The model under review builds one solid part; all positions refer to its coordinate system, in mm. Face numbers are marked on the shaded views. A direction names the side the tool comes from. Round coordinates to 2 decimals unless told otherwise and drop trailing zeros. Write each loop counter-clockwise with the first axis right and the second up, starting at its lowest first coordinate (ties: lowest second). Pieces come first, ordered by that corner, then holes. Notation, with made-up numbers: (86, 16) -> (117, 16) arc R27 ccw to (117, 36) -> close; hole circle Ø1 at (52.25, 34). An arc over 180 degrees is marked (long way). Answer in a Markdown table with one row per item. Add a question column.
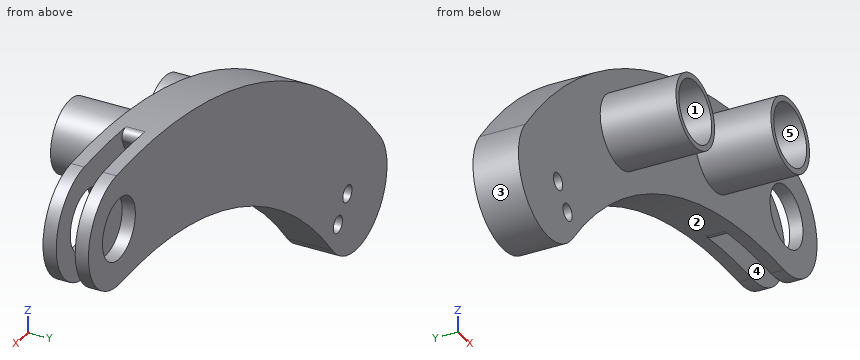
```python
from build123d import *

# Parameters (mm, degrees)
BOSS_EXTRUDE4_DEPTH = 11.999999999999996
BOSS_EXTRUDE5_DEPTH = 3.5
BOSS_EXTRUDE6_DEPTH = 12
CUT_EXTRUDE2_DEPTH  = 8.5
BOSS_EXTRUDE7_DEPTH = 3.5000000000000004
SKETCH2_R           = 8.1
CUT_EXTRUDE3_DEPTH  = 12
FILLET1_R           = 5
FILLET2_R           = 2
SKETCH3_R           = 2.2499999999999964
CUT_EXTRUDE4_DEPTH  = 12
SKETCH4_R           = 9.500000000000002
SKETCH4_R_2         = 8.1
SKETCH4_R_3         = 9.499999999999995
SKETCH4_R_4         = 8.099999999999993
BOSS_EXTRUDE8_DEPTH = 19.999999999999993


with BuildPart() as part:
    # Sketch1 → Boss-Extrude4 (new body)
    with BuildSketch(Plane(origin=(0, 0, 0), x_dir=(1, 0, 0), z_dir=(0, 1, 0))):
        with BuildLine():
            ThreePointArc((-105.23956914411866, 60.05130546378884), (-126.31086817026393, 62.500868149406244), (-128.76043085588134, 41.429569123260976))
            ThreePointArc((-128.76043085588134, 41.42956912326096), (-78.3921989201775, 0.4513014224205847), (-15.424890802752289, -15.400995588922257))
            ThreePointArc((-15.424890802752284, -15.400995588922251), (-20.878753235246265, -0.5691494549701637), (-16.67921047602729, 14.665420305521598))
            ThreePointArc((-16.679210476027265, 14.665420305521593), (-65.8857769449076, 27.74562513419724), (-105.23956914411866, 60.05130546378885))
        make_face()
    extrude(amount=BOSS_EXTRUDE4_DEPTH)

    # Sketch1_6 → Boss-Extrude5 (add)
    with BuildSketch(Plane(origin=(0, 0, 0), x_dir=(1, 0, 0), z_dir=(0, 1, 0))):
        with BuildLine():
            ThreePointArc((-16.67921047602729, 14.665420305521598), (-20.878753235246265, -0.5691494549701637), (-15.424890802752284, -15.400995588922251))
            ThreePointArc((-15.424890802752289, -15.400995588922257), (-7.086372530747029, -15.406529466177687), (1.2395691441186596, -14.94869453621115))
            ThreePointArc((1.2395691441186607, -14.948694536211157), (14.948694536211152, 1.2395691441186514), (-1.2395691441186483, 14.948694536211152))
            ThreePointArc((-1.2395691441186347, 14.94869453621115), (-8.954828429393212, 14.55844291928571), (-16.679210476027265, 14.665420305521593))
        make_face()
    extrude(amount=BOSS_EXTRUDE5_DEPTH)

    # Sketch1_8 → Boss-Extrude6 (add)
    with BuildSketch(Plane(origin=(0, 0, 0), x_dir=(1, 0, 0), z_dir=(0, 1, 0))):
        with BuildLine():
            ThreePointArc((-16.67921047602729, 14.665420305521598), (-20.878753235246265, -0.5691494549701637), (-15.424890802752284, -15.400995588922251))
            ThreePointArc((-15.424890802752289, -15.400995588922257), (-7.086372530747029, -15.406529466177687), (1.2395691441186596, -14.94869453621115))
            ThreePointArc((1.2395691441186607, -14.948694536211157), (14.948694536211152, 1.2395691441186514), (-1.2395691441186483, 14.948694536211152))
            ThreePointArc((-1.2395691441186347, 14.94869453621115), (-8.954828429393212, 14.55844291928571), (-16.679210476027265, 14.665420305521593))
        make_face()
    extrude(amount=BOSS_EXTRUDE6_DEPTH)

    # Sketch1_9 → Cut-Extrude2 (cut)
    with BuildSketch(Plane(origin=(0, 0, 0), x_dir=(1, 0, 0), z_dir=(0, 1, 0))):
        with BuildLine():
            ThreePointArc((-16.67921047602729, 14.665420305521598), (-20.878753235246265, -0.5691494549701637), (-15.424890802752284, -15.400995588922251))
            ThreePointArc((-15.424890802752289, -15.400995588922257), (-7.086372530747029, -15.406529466177687), (1.2395691441186596, -14.94869453621115))
            ThreePointArc((1.2395691441186607, -14.948694536211157), (14.948694536211152, 1.2395691441186514), (-1.2395691441186483, 14.948694536211152))
            ThreePointArc((-1.2395691441186347, 14.94869453621115), (-8.954828429393212, 14.55844291928571), (-16.679210476027265, 14.665420305521593))
        make_face()
    extrude(amount=CUT_EXTRUDE2_DEPTH, mode=Mode.SUBTRACT)

    # Sketch1_10 → Boss-Extrude7 (add)
    with BuildSketch(Plane(origin=(0, 0, 0), x_dir=(1, 0, 0), z_dir=(0, 1, 0))):
        with BuildLine():
            ThreePointArc((-16.67921047602729, 14.665420305521598), (-20.878753235246265, -0.5691494549701637), (-15.424890802752284, -15.400995588922251))
            ThreePointArc((-15.424890802752289, -15.400995588922257), (-7.086372530747029, -15.406529466177687), (1.2395691441186596, -14.94869453621115))
            ThreePointArc((1.2395691441186607, -14.948694536211157), (14.948694536211152, 1.2395691441186514), (-1.2395691441186483, 14.948694536211152))
            ThreePointArc((-1.2395691441186347, 14.94869453621115), (-8.954828429393212, 14.55844291928571), (-16.679210476027265, 14.665420305521593))
        make_face()
    extrude(amount=BOSS_EXTRUDE7_DEPTH)

    # Sketch2 → Cut-Extrude3 (cut)
    with BuildSketch(Plane(origin=(0, 11.999999999999996, 0), x_dir=(1, 0, 0), z_dir=(0, 1, 0))):
        with Locations(Location((0, 0, 0), (0, 0, 270))):
            Circle(SKETCH2_R)
    extrude(amount=-CUT_EXTRUDE3_DEPTH, mode=Mode.SUBTRACT)

    # Fillet1
    fillet1_edges = [part.edges().sort_by_distance(p)[0] for p in [
        (-16.67921047602728, 6, -14.665420305521597),
    ]]
    fillet(fillet1_edges, radius=FILLET1_R)

    # Fillet2
    fillet2_edges = [part.edges().sort_by_distance(p)[0] for p in [
        (-15.424890802752289, 6, 15.400995588922266),
    ]]
    fillet(fillet2_edges, radius=FILLET2_R)

    # Sketch3 → Cut-Extrude4 (cut)
    with BuildSketch(Plane(origin=(0, 11.999999999999996, 0), x_dir=(1, 0, 0), z_dir=(0, 1, 0))):
        with Locations(Location((-107.81660725396851, 54.30249040498051, 0), (0, 0, 270))):
            Circle(SKETCH3_R)
        with Locations(Location((-112.49908312253997, 48.44378579216329, 0), (0, 0, 270))):
            Circle(SKETCH3_R)
    extrude(amount=-CUT_EXTRUDE4_DEPTH, mode=Mode.SUBTRACT)

    # Sketch4 → Boss-Extrude8 (add)
    # profile 1 of 2: a face of its own
    with BuildSketch(Plane(origin=(0, 0, 0), x_dir=(1, 0, 0), z_dir=(0, 1, 0))):
        with Locations(Location((-35.51993478051481, 1.811997227050931, 0), (0, 0, 270))):
            Circle(SKETCH4_R)
        with Locations(Location((-35.51993478051481, 1.811997227050931, 0), (0, 0, 270))):
            Circle(SKETCH4_R_2, mode=Mode.SUBTRACT)
    # profile 2 of 2: a face of its own
    with BuildSketch(Plane(origin=(0, 0, 0), x_dir=(1, 0, 0), z_dir=(0, 1, 0))):
        with Locations(Location((-82.24716798080135, 19.60428986869888, 0), (0, 0, 270))):
            Circle(SKETCH4_R_3)
        with Locations(Location((-82.24716798080135, 19.60428986869888, 0), (0, 0, 270))):
            Circle(SKETCH4_R_4, mode=Mode.SUBTRACT)
    extrude(amount=-BOSS_EXTRUDE8_DEPTH)


solid = part.part
```
1. Tool access review of the marked faces 1 and 2: name each direction out of +Z, -Z, +X, -X, +Y, -Y from which nothing blocks a thin tool from reaching the whole face with its end or side.
2. Add section D-D on x = -85. Write out the cut boundary in (y, z), plus the area to 3 significant figures.
3. Add section A-A on z = 0. Write out the cut boundary in (x, y), plus the area to 3 significant figures.
4. Add section B-B on y = -15. Write out the cut boundary in (x, z).
5. Mouldability with a two-part tool opening along X and no side actions: class the marked faces 3, 4 and 5 as pulls with the +X half, pulls with the -X half, needs draft (parallel to the pull), parting line crosses it, or undercut.
6. For L1, parallel to Y at x = -32.5, z = 10.5; L2, parallel to X at y = -3.5, z = -19; L3, parallel to Z at x = -106, y = 6.5, list the stretches that pass through material, from the lowest coordinate up.
7. Insertion check: pin 1 Ø2 at (x, y) = (-34.5, 0) entering from +Z; pin 2 Ø1.5 at (y, z) = (-7, -29) entering from -X; pin 3 Ø7 at (x, z) = (-107.82, -54.3) entering from +Y; pin 4 Ø15.5 at (x, z) = (-12, -7.5) entering from -Y. Each pin has a flat end and moves straight along its axis. Give the tip position at first contact, or say it passes through.
8. Add section C-C on x = -6.5. Write out the cut boundary in (y, z), plus the area to 3 significant figures.
Filled in:
| question | item | result |
|---|---|---|
| 1 | face 1 | -Y |
| 1 | face 2 | -Z, +Y, -Y |
| 2 | outline | (-20, -28.7) -> (0, -28.7) -> (0, -39.95) -> (12, -39.95) -> (12, -3.97) -> (0, -3.97) -> (0, -10.51) -> (-20, -10.51) -> (-20, -11.99) -> (0, -11.99) -> (0, -27.22) -> (-20, -27.22) -> close |
| 2 | area | 491 mm² |
| 3 | outline | (-77.48, 0) -> (-44.85, 0) -> (-44.85, -20) -> (-43.41, -20) -> (-43.41, 0) -> (-27.63, 0) -> (-27.63, -20) -> (-26.19, -20) -> (-26.19, 0) -> (-8.1, 0) -> (-8.1, 3.5) -> (-20.9, 3.5) -> (-20.9, 8.5) -> (-8.1, 8.5) -> (-8.1, 12) -> (-77.48, 12) -> close; (8.1, 0) -> (15, 0) -> (15, 3.5) -> (8.1, 3.5) -> close; (8.1, 8.5) -> (15, 8.5) -> (15, 12) -> (8.1, 12) -> close |
| 3 | area | 874 mm² |
| 4 | outline | circle Ø19 at (-82.25, -19.6); circle Ø19 at (-35.52, -1.81); hole circle Ø16.2 at (-82.25, -19.6); hole circle Ø16.2 at (-35.52, -1.81) |
| 5 | face 3 | parting line crosses it |
| 5 | face 4 | needs draft |
| 5 | face 5 | undercut |
| 6 | L1 | 0 to 12 |
| 6 | L2 | -91.73 to -90.32, -74.17 to -72.77 |
| 6 | L3 | -60.94 to -55.63, -52.97 to -18.33 |
| 7 | pin 1 | z = 13.79 |
| 7 | pin 2 | x = -86.18 |
| 7 | pin 3 | y = 12 |
| 7 | pin 4 | y = 0 |
| 8 | outline | (0, -14.63) -> (3.5, -14.63) -> (3.5, -4.83) -> (0, -4.83) -> close; (0, 4.83) -> (3.5, 4.83) -> (3.5, 15.39) -> (0, 15.39) -> close; (8.5, -14.63) -> (12, -14.63) -> (12, -4.83) -> (8.5, -4.83) -> close; (8.5, 4.83) -> (12, 4.83) -> (12, 15.39) -> (8.5, 15.39) -> close |
| 8 | area | 142 mm² |
